Check sheet for the modelled part. Datum: model origin and axes. Units: mm. A direction names the side the tool comes from. Give positions to 0.01 mm unless a question says otherwise; leave off trailing zeros. Loops run counter-clockwise (first coordinate to the right, second up) from the corner with the lowest first, then second, coordinate; pieces in that order, holes last. Notation, with made-up numbers: (21, 72.5) -> (28, 72.5) arc R11 ccw to (28, 90.5) -> close; hole circle Ø10 at (-35, -3). An arc over 180 degrees is marked (long way). Write each question's results on one line, items separated by ' | '. Start each with the question number.
Item 1: Cross-section at D-D on x = 18. Enter the section's corners in (y, z) (1 decimal), then the cut area to 3 significant figures.
Item 2: Cross-section at C-C on z = -1. Enter the section's corners in (x, y) (1 decimal).
Item 3: Access from +Z, -Z, +X, -X, +Y, -Y to the whole of each face (thin tool, end or side, straight path). Record for faces 1 (the face through (-25.29, -6.71, 7.03)), 2 (the face through (0, -7.938, -9)), 3 (the face through (18.25, -4.7, -9.34)).
Item 4: Cross-section at A-A on y = -7.25. State how many separate pieces and enclosed holes the cut face has, then the cut area to 3 significant figures.
Item 5: Gauge pin test, flat ends, axial feed: pin 1 Ø4 at (x, y) = (-11, -6.5) entering from +Z; pin 2 Ø9 at (x, z) = (28.58, 1.45) entering from +Y; pin 3 Ø1 at (x, y) = (-30, -2.5) entering from +Z. Record the tip position at first contact, or that the pin passes through.
Item 6: Scan lines: line 1 along X through (y, z) = (-6, 0.5); line 2 along X through (y, z) = (-1.75, 3); line 3 along X through (y, z) = (-6.75, 15.5). Record each from-to range of solid material in increasing order.
Item 7: Mould release check, pull along Z, two halves, no side actions. Record for faces 4 (the face through (-31.77, -6.71, 7.08)), 5 (the face through (-20.369, -4.153, 12.658)), 6 (the face through (31.768, -6.708, -4.188)), 7 (the face through (-13, 1, 15.062)): pulls with the +Z half, pulls with the -Z half, needs draft (parallel to the pull), parting line crosses it, or undercut.
Item 8: Cross-section at B-B on x = 0. Enter the section's corners in (y, z) (1 decimal).
from build123d import *

# Parameters (mm, degrees)
F2_DEPTH = 7.9375
F3_R     = 14.4145
F3_R_2   = 12.7
F4_DEPTH = 1.5875
F5_R     = 4.0005
F6_DEPTH = 5.715
F7_DEPTH = 9.526
F8_DEPTH = 1.3716


with BuildPart() as f2:
    # F1 (on Front) → F2 (new body)
    with BuildSketch(Plane.XZ):
        with BuildLine():
            ThreePointArc((-9.2268886896, 15.0622), (0, 18.4023), (9.2268886896, 15.0622))
            Line((9.2268886896, 15.0622), (16.1826561854, 15.0622))
            ThreePointArc((16.1826561854, 15.0622), (14.8730374451, 16.1166346988), (13.6527661358, 17.2732987427))
            ThreePointArc((13.6527661358, 17.2732987427), (0, 23.0378), (-13.6527661358, 17.2732987427))
            ThreePointArc((-13.6527661358, 17.2732987427), (-14.8730374451, 16.1166346988), (-16.1826561854, 15.0622))
            Line((-16.1826561854, 15.0622), (-9.2268886896, 15.0622))
        make_face()
        with BuildLine():
            ThreePointArc((9.2268886896, 15.0622), (13.0533290249, 10.1024064155), (14.4145, 3.9878))
            ThreePointArc((14.4145, 3.9878), (-6.1146064155, -9.0655290249), (-9.2268886896, 15.0622))
            Line((-9.2268886896, 15.0622), (-16.1826561854, 15.0622))
            ThreePointArc((-16.1826561854, 15.0622), (-22.0501747614, 12.0215629242), (-28.575, 10.9728))
            ThreePointArc((-28.575, 10.9728), (-38.1, 1.4478), (-28.575, -8.0772))
            ThreePointArc((-28.575, -8.0772), (-18.3903131498, -9.3039356127), (-8.7882106244, -12.9139707363))
            ThreePointArc((-8.7882106244, -12.9139707363), (0, -15.0622), (8.7882106244, -12.9139707363))
            ThreePointArc((8.7882106244, -12.9139707363), (18.3903131498, -9.3039356127), (28.575, -8.0772))
            ThreePointArc((28.575, -8.0772), (38.1, 1.4478), (28.575, 10.9728))
            ThreePointArc((28.575, 10.9728), (22.0501747614, 12.0215629242), (16.1826561854, 15.0622))
            Line((16.1826561854, 15.0622), (9.2268886896, 15.0622))
        make_face()
    extrude(amount=F2_DEPTH)

    # F3 (on face) → F4 (join)
    with BuildSketch(Plane.XZ.offset(7.9375)):
        with BuildLine():
            ThreePointArc((28.575, -8.0772), (38.1, 1.4478), (28.575, 10.9728))
            ThreePointArc((28.575, 10.9728), (20.4760903835, 12.6124877504), (13.6527661358, 17.2732987427))
            ThreePointArc((13.6527661358, 17.2732987427), (0, 23.0378), (-13.6527661358, 17.2732987427))
            ThreePointArc((-13.6527661358, 17.2732987427), (-20.4760903835, 12.6124877504), (-28.575, 10.9728))
            ThreePointArc((-28.575, 10.9728), (-38.1, 1.4478), (-28.575, -8.0772))
            ThreePointArc((-28.575, -8.0772), (-18.3903131498, -9.3039356127), (-8.7882106244, -12.9139707363))
            ThreePointArc((-8.7882106244, -12.9139707363), (0, -15.0622), (8.7882106244, -12.9139707363))
            ThreePointArc((8.7882106244, -12.9139707363), (18.3903131498, -9.3039356127), (28.575, -8.0772))
        make_face()
        with Locations((0, 3.9878)):
            Circle(F3_R, mode=Mode.SUBTRACT)
        with Locations((0, 3.9878)):
            Circle(F3_R)
        with Locations((0, 3.9878)):
            Circle(F3_R_2, mode=Mode.SUBTRACT)
    extrude(amount=F4_DEPTH)

    # F5 (on face) → F6 (cut)
    with BuildSketch(Plane.XZ.offset(9.525)):
        Polygon((-22.098, -2.2916976935), (-22.098, 5.1872976935), (-28.575, 8.9267953871), (-35.052, 5.1872976935), (-35.052, -2.2916976935), (-28.575, -6.0311953871), align=None)
        with Locations((-28.575, 1.4478)):
            Circle(F5_R, mode=Mode.SUBTRACT)
        Polygon((22.098, 5.1872976935), (22.098, -2.2916976935), (28.575, -6.0311953871), (35.052, -2.2916976935), (35.052, 5.1872976935), (28.575, 8.9267953871), align=None)
        with Locations((28.575, 1.4478)):
            Circle(F5_R, mode=Mode.SUBTRACT)
    extrude(amount=-F6_DEPTH, mode=Mode.SUBTRACT)

    # F7 (cut, through all): faces of the model
    f7_faces = [f2.faces().sort_by_distance(p)[0] for p in [
        (-28.575, -9.525, 1.4478),
        (28.575, -9.525, 1.4478),
    ]]
    extrude(f7_faces, amount=-F7_DEPTH, mode=Mode.SUBTRACT)

    # F1 (on Front) → F8 (join)
    with BuildSketch(Plane.XZ):
        with BuildLine():
            ThreePointArc((-9.2268886896, 15.0622), (0, 18.4023), (9.2268886896, 15.0622))
            Line((9.2268886896, 15.0622), (16.1826561854, 15.0622))
            ThreePointArc((16.1826561854, 15.0622), (14.8730374451, 16.1166346988), (13.6527661358, 17.2732987427))
            ThreePointArc((13.6527661358, 17.2732987427), (0, 23.0378), (-13.6527661358, 17.2732987427))
            ThreePointArc((-13.6527661358, 17.2732987427), (-14.8730374451, 16.1166346988), (-16.1826561854, 15.0622))
            Line((-16.1826561854, 15.0622), (-9.2268886896, 15.0622))
        make_face()
    extrude(amount=-F8_DEPTH)


solid = f2.part
Answer sheet:
1) outline: (-9.5, -9.4) -> (0, -9.4) -> (0, 13.9) -> (-9.5, 13.9) -> close | area: 222 mm²
2) outline: (-37.8, -9.5) -> (-35.1, -9.5) -> (-35.1, -3.8) -> (-31.7, -3.8) -> (-31.7, 0) -> (-37.8, 0) -> close; (-25.4, -3.8) -> (-22.1, -3.8) -> (-22.1, -9.5) -> (-11.7, -9.5) -> (-11.7, -7.9) -> (-13.5, -7.9) -> (-13.5, 0) -> (-25.4, 0) -> close; (11.7, -9.5) -> (22.1, -9.5) -> (22.1, -3.8) -> (25.4, -3.8) -> (25.4, 0) -> (13.5, 0) -> (13.5, -7.9) -> (11.7, -7.9) -> close; (31.7, -3.8) -> (35.1, -3.8) -> (35.1, -9.5) -> (37.8, -9.5) -> (37.8, 0) -> (31.7, 0) -> close
3) face 1: -Y | face 2: +Y | face 3: -Z, +X, +Y, -Y
4) separate pieces: 1 | enclosed holes: 3 | area: 942 mm²
5) pin 1: stops at z = 20.78 | pin 2: stops at y = 0 | pin 3: stops at z = 10.93
6) line 1: x = -38.05 to -35.05, -22.1 to -13.99, 13.99 to 22.1, 35.05 to 38.05 | line 2: x = -37.97 to -32.26, -24.89 to -14.38, 14.38 to 24.89, 32.26 to 37.97 | line 3: x = -15.61 to -8.67, 8.67 to 15.61
7) face 4: undercut | face 5: pulls with the +Z half | face 6: undercut | face 7: pulls with the -Z half
8) outline: (-9.5, -15.1) -> (0, -15.1) -> (0, -10.4) -> (-7.9, -10.4) -> (-7.9, -8.7) -> (-9.5, -8.7) -> close; (-9.5, 16.7) -> (-7.9, 16.7) -> (-7.9, 18.4) -> (1.4, 18.4) -> (1.4, 23) -> (-9.5, 23) -> close
